CAD build for the part. Positions are in the model's coordinates, mm. A direction names the side the tool comes from. Round coordinates to 2 decimals unless told otherwise and drop trailing zeros. Loops run counter-clockwise (first coordinate to the right, second up) from the corner with the lowest first, then second, coordinate; pieces in that order, holes last. Notation, with made-up numbers: (84, 75) - (142, 75) arc R17 cw to (142, 84) - close; hole circle Ø3 at (63, -19.5). An arc over 180 degrees is marked (long way). Use one line per item in the form item = value.
Autodesk Inventor part; units mm, degrees
ref_plane "YZ Plane" through (0, 0, 0) normal (1, 0, 0) x (0, 1, 0)
ref_plane "XZ Plane" through (0, 0, 0) normal (0, 1, 0) x (-1, 0, 0)
ref_plane "XY Plane" through (0, 0, 0) normal (0, 0, 1) x (1, 0, 0)
sketch "Sketch1" plane through (0, 0, 0) normal (0, 1, 0) x (-1, 0, 0)
  arc A0 (0, -490) -> (-342.9286, 350) centre (0, 0) ccw
  line L0 (0, -490) -> (-650, -490)
  line L1 (-650, -490) -> (-650, 350)
  line L2 (-650, 350) -> (-342.9286, 350)
  dimension "d1" = 980
  dimension "d2" = 350
  dimension "d3" = 650
extrude "Extrusion1" add sketch "Sketch1" along normal mid plane 16
sketch "Sketch2" plane through (0, 8, 0) normal (0, 1, 0) x (1, 0, 0)
  arc A0 (0, 490) -> (342.9286, -350) centre (0, 0) ccw
  line L0 (650, -350) -> (650, 490)
  line L1 (650, 490) -> (0, 490)
  line L2 (435, 465) -> (525, 465)
  line L3 (530, 460) -> (530, 445)
  line L4 (525, 440) -> (435, 440)
  line L5 (430, 445) -> (430, 460)
  arc A1 (435, 465) -> (430, 460) centre (435, 460) ccw
  arc A2 (430, 445) -> (435, 440) centre (435, 445) ccw
  arc A3 (525, 440) -> (530, 445) centre (525, 445) ccw
  arc A4 (530, 460) -> (525, 465) centre (525, 460) ccw
  line L6 (0, 0) -> (-346.4823, 346.4823) construction
  line L7 (-289.9138, 353.5534) -> (-353.5534, 289.9138)
  line L8 (-353.5534, 282.8427) -> (-342.9468, 272.2361)
  line L9 (-335.8757, 272.2361) -> (-272.2361, 335.8757)
  line L10 (-272.2361, 342.9468) -> (-282.8427, 353.5534)
  arc A5 (-353.5534, 289.9138) -> (-353.5534, 282.8427) centre (-350.0179, 286.3782) ccw
  arc A6 (-342.9468, 272.2361) -> (-335.8757, 272.2361) centre (-339.4113, 275.7716) ccw
  arc A7 (-272.2361, 335.8757) -> (-272.2361, 342.9468) centre (-275.7716, 339.4113) ccw
  arc A8 (-282.8427, 353.5534) -> (-289.9138, 353.5534) centre (-286.3782, 350.0179) ccw
  point P0 (430, 465)
  point P1 (530, 465)
  point P2 (430, 440)
  dimension "d6" = 100
  dimension "d7" = 25
  dimension "d8" = 25
  dimension "d9" = 120
  dimension "d10" = 5
  dimension "d11" = 45
  dimension "d15" = 25
  dimension "d16" = 100
  dimension "d17" = 430
  dimension "d18" = 90
  dimension "d19" = 5
extrude "Extrusion2" cut sketch "Sketch2" against normal through all
sketch "Sketch3" plane through (0, 8, 0) normal (0, 1, 0) x (1, 0, 0)
  circle A0 centre (610, 470) radius 4
  circle A1 centre (610, -330) radius 4
  circle A2 centre (610, 70) radius 4
  circle A3 centre (610, 470) radius 2.75
  circle A4 centre (610, 70) radius 2.75
  circle A5 centre (610, -330) radius 2.75
  dimension "d22" = 8
extrude "Extrusion3" cut sketch "Sketch3" against normal through all contours A0 | A1 | A2 | A3 | A4 | A5
ref_plane "Work Plane1" through (0, 0, 0) normal (-0.7071, 0, -0.7071) x (-0.7071, 0, 0.7071)
ref_plane "Work Plane2" through (500, 8, 350) normal (1, 0, 0) x (0, 0, -1)
ref_plane "Work Plane3" through (342.9286, 8, 180) normal (0, 0, 1) x (1, 0, 0)
sketch "Sketch4" plane through (0, 8, 0) normal (0, 1, 0) x (1, 0, 0)
  arc A0 (0, 490) -> (342.9286, -350) centre (0, 0) ccw
  line L0 (-380, -100) -> (-380, 100) construction
  line L1 (-100, 380) -> (100, 380) construction
  line L2 (380, 100) -> (380, -100) construction
  line L3 (100, -380) -> (-100, -380) construction
  line L4 (-15, -385) -> (15, -385)
  line L5 (15, -385) -> (15, -395)
  line L6 (15, -395) -> (-15, -395)
  line L7 (-15, -395) -> (-15, -385)
  line L8 (-395, 15) -> (-385, 15)
  line L9 (-385, 15) -> (-385, -15)
  line L10 (-385, -15) -> (-395, -15)
  line L11 (-395, -15) -> (-395, 15)
  line L12 (-15, 395) -> (15, 395)
  line L13 (15, 395) -> (15, 385)
  line L14 (15, 385) -> (-15, 385)
  line L15 (-15, 385) -> (-15, 395)
  line L16 (385, 15) -> (395, 15)
  line L17 (395, 15) -> (395, -15)
  line L18 (395, -15) -> (385, -15)
  line L19 (385, -15) -> (385, 15)
  line L20 (0, 0) -> (-490, 0) construction
  line L21 (0, 0) -> (0, 490) construction
  dimension "d27" = 5
  dimension "d28" = 5
  dimension "d29" = 10
  dimension "d30" = 30
extrude "Extrusion4" cut sketch "Sketch4" against normal blind 8
properties part number "Base_Left" material "MDF Medium Density Fiberboard"
1) Two-plate mould, pull along X, no slides. Class faces 1 (the flat face through (88, -8, 7)), 2 (the flat face through (-321.29, 0.11, -322.18)), 3 (the cylindrical face through (-448.404, -0.112, 197.569)): +X half, -X half, draft (parallel to the pull), parting line (faces both ways), or undercut.
Report:
face_1 = draft
face_2 = undercut
face_3 = parting line
2) Drill centre lines: probe 1 along Z at (x, y) = (610, -0.5); probe 2 along Z at (x, y) = (474, 1.5); probe 3 along X at (y, z) = (0.5, -70). Where is each one in solid material? Low to high.
Report:
probe_1 = -490 to -474, -466 to -74, -66 to 326, 334 to 350
probe_2 = -490 to -465, -440 to 350
probe_3 = -484.97 to 606, 614 to 650
3) Slice it at A-A (y = -4). Write the cut outline in (x, z), plus the area to 3 significant figures.
Report:
outline = (0, -490) - (650, -490) - (650, 350) - (342.93, 350) arc R490 ccw (long way) to start; hole (-353.55, -289.91) - (-289.91, -353.55) arc R5 ccw to (-282.84, -353.55) - (-272.24, -342.95) arc R5 ccw to (-272.24, -335.88) - (-335.88, -272.24) arc R5 ccw to (-342.95, -272.24) - (-353.55, -282.84) arc R5 ccw to start; hole (430, -460) arc R5 ccw to (435, -465) - (525, -465) arc R5 ccw to (530, -460) - (530, -445) arc R5 ccw to (525, -440) - (435, -440) arc R5 ccw to (430, -445) - close; hole circle Ø8 at (610, -470); hole circle Ø8 at (610, -70); hole circle Ø8 at (610, 330)
area = 951,000 mm^2
4) Slice it at C-C (x = -111.5). Write the cut outline in (y, z), plus the area to 3 significant figures.
Report:
outline = (-8, -477.15) - (8, -477.15) - (8, 477.15) - (-8, 477.15) - close
area = 15,300 mm^2
5) Slice it at B-B (z = -162). Write the cut outline in (x, y).
Report:
outline = (-462.45, -8) - (650, -8) - (650, 8) - (-462.45, 8) - close
6) Flat gauge pins, fed straight in: pin 1 (2.5 mm diameter, centred on y = 4, z = 391.5, fed in from -X); pin 2 (4 mm diameter, centred on x = 390, y = 3.5, fed in from +Z); pin 3 (2.5 mm diameter, centred on y = 3, z = 389, fed in from +X). Where does each tip first touch, or does it go through?
Report:
pin_1 = -296.32
pin_2 = 350
pin_3 = 299.58
7) Tool access for faces 4 (the flat face through (88, 8, 7)), 5 (the flat face through (-304.5, 0.11, -303.61)): list every direction of +Z, -Z, +X, -X, +Y, -Y with a clear straight run to the whole face (end or side of a thin tool).
Report:
face_4 = +Z, -Z, +X, -X, +Y
face_5 = +Y, -Y
